Answer from the drawing. Dimensions are ordinates in mm from the lowest x, y and z of the part. A direction names the side the tool comes from. Coordinates: 2 decimals unless noted, no trailing zeros. Loops run counter-clockwise (first coordinate to the right, second up) from the corner with the lowest first, then second, coordinate; pieces in that order, holes last. Notation, with made-up numbers: M 40,62 L 73,62 A26 cw 73,99 Z; hole C -7.75,-21.75 d4. An arc over 180 degrees is marked long. Put each result on its own line as item: value.
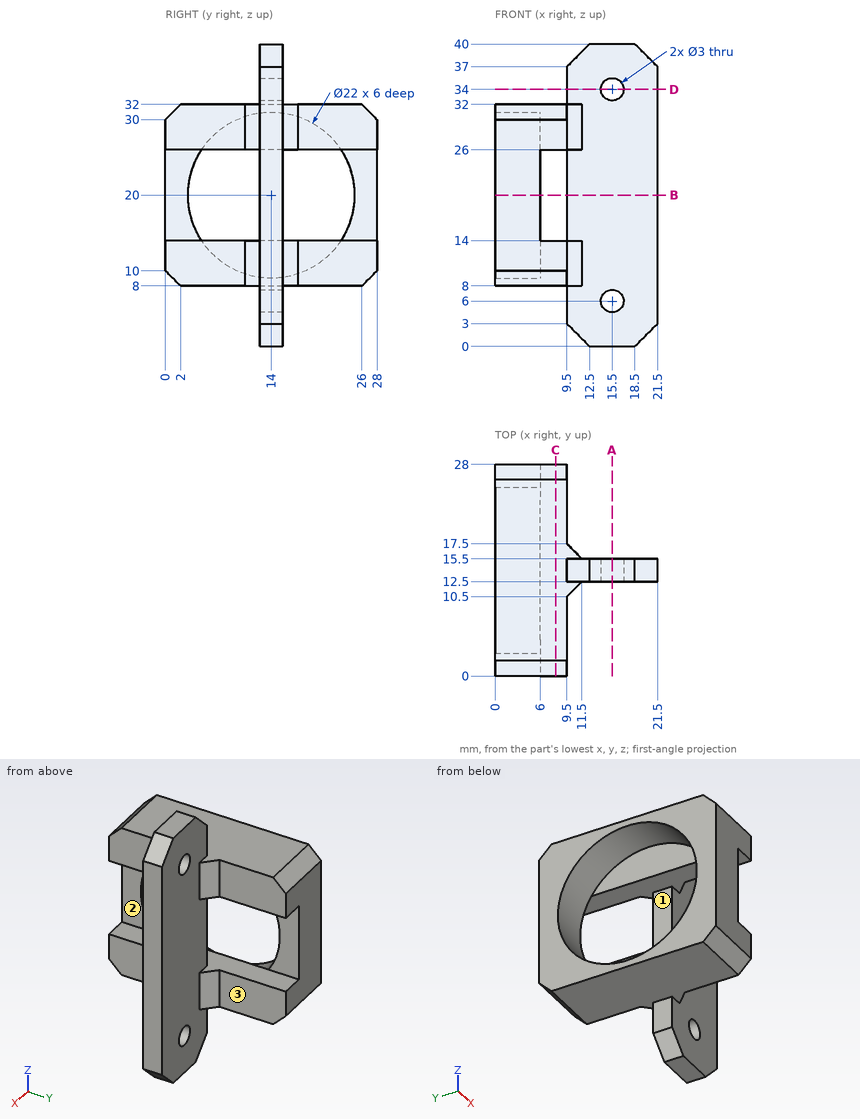
1) Find section C-C, the plane x = 8. Write down the section's boundary in (y, z), plus the area to 3 significant figures.
Answer list:
outline: M 0,10 L 2,8 L 26,8 L 28,10 L 28,14 L 0,14 Z; M 0,26 L 28,26 L 28,30 L 26,32 L 2,32 L 0,30 Z
area: 328 mm^2
2) Find section B-B, the plane z = 20. Write down the section's boundary in (x, y).
Answer list:
outline: M 0,0 L 6,0 L 6,3 L 0,3 Z; M 0,25 L 6,25 L 6,28 L 0,28 Z; M 9.5,12.5 L 21.5,12.5 L 21.5,15.5 L 9.5,15.5 Z
3) Find section D-D, the plane z = 34. Write down the section's boundary in (x, y), plus the area to 3 significant figures.
Answer list:
outline: M 9.5,12.5 L 14,12.5 L 14,15.5 L 9.5,15.5 Z; M 17,12.5 L 21.5,12.5 L 21.5,15.5 L 17,15.5 Z
area: 27.0 mm^2
4) Which of the six approach directions +Z, -Z, +X, -X, +Y, -Y give full straight-line access (tool end or side, diameter ignored) to the marked faces 1, 2 and 3?
Answer list:
face 1: -X, +Y, -Y
face 2: +X, +Y, -Y
face 3: +Z, -Z, +X, +Y
5) Find section A-A, the plane x = 15.5. Write down the section's boundary in (y, z), plus the area to 3 significant figures.
Answer list:
outline: M 12.5,0 L 15.5,0 L 15.5,4.5 L 12.5,4.5 Z; M 12.5,7.5 L 15.5,7.5 L 15.5,32.5 L 12.5,32.5 Z; M 12.5,35.5 L 15.5,35.5 L 15.5,40 L 12.5,40 Z
area: 102 mm^2
6) Straight lines are drawn through the part: line 1 (Z direction, x = 9.25, y = 7.5); line 2 (Z direction, x = 2, y = 14); line 3 (Y direction, x = 10.5, z = 7.5). For each, find the intervals that lie inside material, in ascending order. Write a range as [from, to].
Answer list:
line 1: z = [8, 14], [26, 32]
line 2: z = [8, 9], [31, 32]
line 3: y = [12.5, 15.5]
7) Given pin 1 Ø4 at (y, z) = (24.5, 17.5) entering from +X; pin 2 Ø0.9 at (y, z) = (14, 34) entering from -X; pin 3 Ø3 at (y, z) = (24.5, 5.5) entering from +X; pin 4 Ø6.5 at (y, z) = (5, 28.5) entering from +X, each flat-ended and moving along its own axis, determine where each tip first touches the part or whether it passes through.
Answer list:
pin 1: stops at x = 6
pin 2: stops at x = 9.5
pin 3: passes through
pin 4: stops at x = 9.5
